from build123d import *

# Parameters (mm, degrees)
SKETCH1_W                = 54.212076584
SKETCH1_H                = 45
SKETCH1_R                = 10
SKETCH1_R_2              = 1.575
BOSS_EXTRUDE1_DEPTH      = 5
BOSS_EXTRUDE2_DEPTH      = 50
BOSS_EXTRUDE2_DEPTH_BACK = 5
SKETCH2_W                = 54.212076584
SKETCH2_H                = 5
FILLET3_R                = 4


with BuildPart() as part:
    # Sketch1 → Boss-Extrude1 (new body)
    with BuildSketch(Plane.XY):
        Rectangle(SKETCH1_W, SKETCH1_H)
        Circle(SKETCH1_R, mode=Mode.SUBTRACT)
        with Locations((0, 14)):
            Circle(SKETCH1_R_2, mode=Mode.SUBTRACT)
        with Locations((12.124355653, -7)):
            Circle(SKETCH1_R_2, mode=Mode.SUBTRACT)
        with Locations((-12.124355653, -7)):
            Circle(SKETCH1_R_2, mode=Mode.SUBTRACT)
    extrude(amount=BOSS_EXTRUDE1_DEPTH)

    # Sketch2 → Boss-Extrude2 (add, two sides: drawn at the far end of the back side and taken through both)
    with BuildSketch(Plane(origin=(0, 0, 0), x_dir=(-1, 0, 0), z_dir=(0, 0, -1)).offset(-BOSS_EXTRUDE2_DEPTH_BACK)):
        with Locations((0, -25)):
            Rectangle(SKETCH2_W, SKETCH2_H)
    extrude(amount=BOSS_EXTRUDE2_DEPTH + BOSS_EXTRUDE2_DEPTH_BACK)

    # Fillet3
    fillet3_edges = [part.edges().sort_by_distance(p)[0] for p in [
        (0, -27.5, 5),
        (27.106038292, -25, -50),
        (-27.106038292, -25, -50),
        (0, -22.5, 0),
        (-27.106038292, 22.5, 2.5),
        (27.106038292, 22.5, 2.5),
    ]]
    fillet(fillet3_edges, radius=FILLET3_R)


solid = part.part
Source: CAD feature listing. Evaluate the final solid. Frame: model axes, mm. A direction names the side the tool comes from. Round coordinates to 2 decimals unless told otherwise and drop trailing zeros. Order: outer loops, then holes, each group sorted by start corner. A loop starts at its lowest first (then second) coordinate and runs counter-clockwise, first axis right, second up. Notation, with made-up numbers: (30, 11.25) - (37, 11.25) arc R20 ccw to (37, 41.25) - close; hole circle Ø3 at (74, 31). An arc over 180 degrees is marked (long way). Use a Markdown table: item, result. Add a question column.
1. Set-up query: faces 4 (the flat face through (-27.106, -23, -11)), 5 (the flat face through (0, -22.5, -27)). Return all of +Z, -Z, +X, -X, +Y, -Y with unobstructed straight access to the full face (end or side cutting, diameter ignored); none if empty.
2. Line query: probe 1 along Y at (x, z) = (0, 3) (3 decimals); probe 2 along Y at (x, z) = (7.5, -17.5); probe 3 along Z at (x, y) = (-2.5, 11.5). Output: solid intervals per line, ascending.
3. Section query C-C (x = 6.5). Return the cut outline in (y, z).
4. Section query B-B (x = 0). Return the cut outline in (y, z) (3 decimals).
5. Section query D-D (x = -16). Return the cut outline in (y, z), then the cut area to 3 significant figures.
6. Mould query, pull axis Y, two halves, no side actions, for faces 1 (the cylindrical face through (11.92, -5.44, 2.46)), 2 (the flat face through (0, -27.5, -24)), 3 (the cylindrical face through (25.965, -24.965, -48.797)). Classes: +Y half, -Y half, draft (parallel to the pull), parting line (faces both ways), or undercut.
7. First-contact query: pin 1 (12 mm diameter, centred on x = 7.5, y = 12, fed in from -Z); pin 2 (10 mm diameter, centred on x = -3, z = -11, fed in from +Y); pin 3 (4 mm diameter, centred on x = -12.12, y = -7, fed in from +Z). Flat tips, straight axial feed; report the tip coordinate or a pass-through.
8. Section query A-A (y = 14). Return the cut outline in (x, z) (3 decimals), then the cut area to 3 significant figures.
Derived:
| question | item | result |
|---|---|---|
| 1 | face 4 | +Z, -Z, -X, +Y, -Y |
| 1 | face 5 | -Z, +X, -X, +Y |
| 2 | probe 1 | -26.964 to -10, 10 to 12.425, 15.575 to 22.5 |
| 2 | probe 2 | -27.5 to -22.5 |
| 2 | probe 3 | 0 to 5 |
| 3 | outline | (-27.5, -50) - (-22.5, -50) - (-22.5, -4) arc R4 cw to (-18.5, 0) - (-7.6, 0) - (-7.6, 5) - (-23.5, 5) arc R4 ccw to (-27.5, 1) - close; (7.6, 0) - (22.5, 0) - (22.5, 5) - (7.6, 5) - close |
| 4 | outline | (-27.5, -50) - (-22.5, -50) - (-22.5, -4) arc R4 cw to (-18.5, 0) - (-10, 0) - (-10, 5) - (-23.5, 5) arc R4 ccw to (-27.5, 1) - close; (10, 0) - (12.425, 0) - (12.425, 5) - (10, 5) - close; (15.575, 0) - (22.5, 0) - (22.5, 5) - (15.575, 5) - close |
| 5 | outline | (-27.5, -50) - (-22.5, -50) - (-22.5, -4) arc R4 cw to (-18.5, 0) - (22.5, 0) - (22.5, 5) - (-23.5, 5) arc R4 ccw to (-27.5, 1) - close |
| 5 | area | 500 mm2 |
| 6 | face 1 | undercut |
| 6 | face 2 | -Y half |
| 6 | face 3 | draft |
| 7 | pin 1 | z = 0 |
| 7 | pin 2 | y = -22.5 |
| 7 | pin 3 | z = 5 |
| 8 | outline | (-27.106, 0) - (-1.575, 0) - (-1.575, 5) - (-27.106, 5) - close; (1.575, 0) - (27.106, 0) - (27.106, 5) - (1.575, 5) - close |
| 8 | area | 255 mm2 |
